from build123d import *

# Parameters (mm, degrees)
F0_W     = 244.475
F0_H     = 12.7
F0_W_2   = 311.15
F0_W_3   = 295.275
F1_DEPTH = 635
F2_W     = 901.7
F2_H     = 685.8
F3_DEPTH = 12.7


with BuildPart() as f1:
    # F0 (on Front) → F1 (new body)
    with BuildSketch(Plane.XZ):
        Polygon((-450.85, 657.225), (-450.85, 9.525), (-438.15, 9.525), (-438.15, 441.325), (-438.15, 454.025), (-438.15, 657.225), align=None)
        Polygon((438.15, 657.225), (450.85, 657.225), (450.85, 676.275), (-450.85, 676.275), (-450.85, 657.225), (-438.15, 657.225), (-193.675, 657.225), (-180.975, 657.225), (130.175, 657.225), (142.875, 657.225), align=None)
        Polygon((-193.675, 9.525), (-180.975, 9.525), (-180.975, 352.425), (-180.975, 365.125), (-180.975, 657.225), (-193.675, 657.225), (-193.675, 454.025), (-193.675, 441.325), align=None)
        with Locations((-315.9125, 447.675)):
            Rectangle(F0_W, F0_H)
        with Locations((-25.4, 358.775)):
            Rectangle(F0_W_2, F0_H)
        Polygon((130.175, 9.525), (142.875, 9.525), (142.875, 307.975), (142.875, 320.675), (142.875, 657.225), (130.175, 657.225), (130.175, 365.125), (130.175, 352.425), align=None)
        with Locations((290.5125, 314.325)):
            Rectangle(F0_W_3, F0_H)
        Polygon((438.15, 9.525), (450.85, 9.525), (450.85, 657.225), (438.15, 657.225), (438.15, 320.675), (438.15, 307.975), align=None)
        Polygon((450.85, -9.525), (450.85, 9.525), (438.15, 9.525), (142.875, 9.525), (130.175, 9.525), (-180.975, 9.525), (-193.675, 9.525), (-438.15, 9.525), (-450.85, 9.525), (-450.85, -9.525), align=None)
    extrude(amount=F1_DEPTH)

    # F2 (on face) → F3 (join)
    with BuildSketch(Plane(origin=(0, 0, 0), x_dir=(-1, 0, 0), z_dir=(0, 1, 0))):
        with Locations((0, 333.375)):
            Rectangle(F2_W, F2_H)
    extrude(amount=F3_DEPTH)


solid = f1.part
The listing builds one solid part. Answer for the finished solid, in the listing's coordinates (mm). Give positions to 0.01 mm unless a question says otherwise; leave off trailing zeros. Order: outer loops, then holes, each group sorted by start corner. A loop starts at its lowest first (then second) coordinate and runs counter-clockwise, first axis right, second up. Notation, with made-up numbers: (64, 89.25) - (88, 89.25) arc R33 ccw to (88, 127.25) - close; hole circle Ø11 at (-23.75, 84). An arc over 180 degrees is marked (long way). One line per item, written item: value. Start each with the question number.
1) Find the intervals of material crossed by L1, parallel to Z at x = 11, y = -279 (3 decimals); L2, parallel to Z at x = -380, y = -28 (3 decimals); L3, parallel to X at y = -468.5, z = 58 (3 decimals), in increasing order.
2) A cutting plane is placed at A-A on z = 244. Give the vertices of the cut face in (x, y) (3 decimals), then the cut area to 3 significant figures.
3) A cutting plane is placed at B-B on y = -90.5. Give the vertices of the cut face in (x, z) (3 decimals), then the cut area to 3 significant figures.
4) Given pin 1 Ø12 at (x, z) = (-225.5, 75) entering from -Y, flat-ended and moving along its own axis, determine where the tip first touches the part or whether it passes through.
5) The mould has two halves that part along X. Classify faces 1 (the face through (450.85, -316, 329)), 2 (the face through (-28, -313, 352.425)), 3 (the face through (-314, 0, 557)), 4 (the face through (6, -316, -9.525)): released by +X, released by -X, zero draft, split by the parting line, or undercut.
6) A cutting plane is placed at C-C on x = -70. Give the vertices of the cut face in (y, z) (3 decimals), then the cut area to 3 significant figures.
Answer sheet:
1. L1: z = -9.525 to 9.525, 352.425 to 365.125, 657.225 to 676.275
1. L2: z = -9.525 to 9.525, 441.325 to 454.025, 657.225 to 676.275
1. L3: x = -450.85 to -438.15, -193.675 to -180.975, 130.175 to 142.875, 438.15 to 450.85
2. outline: (-450.85, -635) - (-438.15, -635) - (-438.15, 0) - (-193.675, 0) - (-193.675, -635) - (-180.975, -635) - (-180.975, 0) - (130.175, 0) - (130.175, -635) - (142.875, -635) - (142.875, 0) - (438.15, 0) - (438.15, -635) - (450.85, -635) - (450.85, 12.7) - (-450.85, 12.7) - close
2. area: 43,700 mm2
3. outline: (-450.85, -9.525) - (450.85, -9.525) - (450.85, 676.275) - (-450.85, 676.275) - close; hole (-438.15, 9.525) - (-193.675, 9.525) - (-193.675, 441.325) - (-438.15, 441.325) - close; hole (-438.15, 454.025) - (-193.675, 454.025) - (-193.675, 657.225) - (-438.15, 657.225) - close; hole (-180.975, 9.525) - (130.175, 9.525) - (130.175, 352.425) - (-180.975, 352.425) - close; hole (-180.975, 365.125) - (130.175, 365.125) - (130.175, 657.225) - (-180.975, 657.225) - close; hole (142.875, 9.525) - (438.15, 9.525) - (438.15, 307.975) - (142.875, 307.975) - close; hole (142.875, 320.675) - (438.15, 320.675) - (438.15, 657.225) - (142.875, 657.225) - close
3. area: 78,100 mm2
4. pin 1: stops at y = 0
5. face 1: released by +X
5. face 2: undercut
5. face 3: undercut
5. face 4: zero draft
6. outline: (-635, -9.525) - (12.7, -9.525) - (12.7, 676.275) - (-635, 676.275) - (-635, 657.225) - (0, 657.225) - (0, 365.125) - (-635, 365.125) - (-635, 352.425) - (0, 352.425) - (0, 9.525) - (-635, 9.525) - close
6. area: 41,000 mm2
